from build123d import *

# Parameters (mm, degrees)
F1_DEPTH = 76.2
F0_W     = 25.4
F0_H     = 126.830346
F2_DEPTH = 12.7
F3_R     = 6.35
F4_DEPTH = 12.7


with BuildPart() as f1:
    # F0 (on Front) → F1 (new body, symmetric)
    with BuildSketch(Plane.XZ):
        Polygon((12.7, 76.030346), (-12.7, 76.030346), (-76.2, 76.030346), (-76.2, 50.630346), (-12.7, 50.630346), (12.7, 50.630346), (76.2, 50.630346), (76.2, 76.030346), align=None)
    extrude(amount=F1_DEPTH, both=True)

    # F0 (on Front) → F2 (join, symmetric)
    with BuildSketch(Plane.XZ):
        with Locations((0, -12.784827)):
            Rectangle(F0_W, F0_H)
    extrude(amount=F2_DEPTH, both=True)

    # F3 (on face) → F4 (cut)
    with BuildSketch(Plane(origin=(-76.2, 0, 0), x_dir=(0, -1, 0), z_dir=(-1, 0, 0))):
        with Locations((31.75, 63.330346)):
            Circle(F3_R)
        with Locations((-31.75, 63.330346)):
            Circle(F3_R)
    extrude(amount=-F4_DEPTH, mode=Mode.SUBTRACT)


solid = f1.part
Can you work these out from the model? Positions are in its coordinate system, mm. A direction names the side the tool comes from. Coordinates: 2 decimals unless noted, no trailing zeros. Write each loop counter-clockwise with the first axis right and the second up, starting at its lowest first coordinate (ties: lowest second). Pieces come first, ordered by that corner, then holes. Notation, with made-up numbers: (-21.5, 20) -> (-13.5, 20) arc R23 cw to (-13.5, 42) -> close; hole circle Ø3 at (16, 58). An arc over 180 degrees is marked (long way). Write item = value, one per line.
(1) Imagine slicing it at B-B (y = -31.75). Please give me the cut outline in (x, z).
Verdict:
outline = (-76.2, 50.63) -> (76.2, 50.63) -> (76.2, 76.03) -> (-76.2, 76.03) -> (-76.2, 69.68) -> (-63.5, 69.68) -> (-63.5, 56.98) -> (-76.2, 56.98) -> close
(2) Thinking about a two-plate mould opening in Y: for faces 4 (the face through (-1, -76.2, 64)), 5 (the face through (76.2, -1, 63)), 6 (the face through (-69.939, 28.82, 57.697)), which applies, +Y half, -Y half, draft (parallel to the pull), parting line (faces both ways), or undercut?
Verdict:
face_4 = -Y half
face_5 = draft
face_6 = undercut
(3) Imagine slicing it at C-C (z = 3). Please give me the cut outline in (x, y).
Verdict:
outline = (-12.7, -12.7) -> (12.7, -12.7) -> (12.7, 12.7) -> (-12.7, 12.7) -> close
(4) Imagine slicing it at A-A (y = -1.5). Please give me the cut outline in (x, z), and give its area (3 significant figures).
Verdict:
outline = (-76.2, 50.63) -> (-12.7, 50.63) -> (-12.7, -76.2) -> (12.7, -76.2) -> (12.7, 50.63) -> (76.2, 50.63) -> (76.2, 76.03) -> (-76.2, 76.03) -> close
area = 7,090 mm^2
(5) Imagine slicing it at D-D (x = 52.5). Please give me the cut outline in (y, z), and give its area (3 significant figures).
Verdict:
outline = (-76.2, 50.63) -> (76.2, 50.63) -> (76.2, 76.03) -> (-76.2, 76.03) -> close
area = 3,870 mm^2
(6) On a 3-axis mill with a long thin cutter (end or side, diameter ignored), from which of +Z, -Z, +X, -X, +Y, -Y can I reach the whole of each face in a straight line? I mean faces 1 (the face through (-12.7, 0, -14)), 2 (the face through (-69.939, -34.68, 57.697)), 3 (the face through (12.7, 0, -14)). Say none if no direction works.
Verdict:
face_1 = -Z, -X, +Y, -Y
face_2 = -X
face_3 = -Z, +X, +Y, -Y
(7) If I drill on probe 1 along Z at (x, y) = (-69, -31); probe 2 along Z at (x, y) = (-70, 31.75); probe 3 along Z at (x, y) = (25.5, 64), over which ranges is the centre line in solid material (lowest first)?
Verdict:
probe_1 = 50.63 to 57.02, 69.64 to 76.03
probe_2 = 50.63 to 56.98, 69.68 to 76.03
probe_3 = 50.63 to 76.03
(8) For pin 1 (14 mm diameter, centred on y = 33, z = 64.5, fed in from -X); pin 2 (4 mm diameter, centred on x = 13.5, y = -33, fed in from -Z); pin 3 (7.5 mm diameter, centred on x = 5, z = -3.5, fed in from +Y); pin 4 (6.5 mm diameter, centred on y = -29, z = 62, fed in from -X), each with a flat end and sliding along its axis, tell me the tip position at first contact or that it passes through.
Verdict:
pin_1 = -76.2
pin_2 = 50.63
pin_3 = 12.7
pin_4 = -63.5
